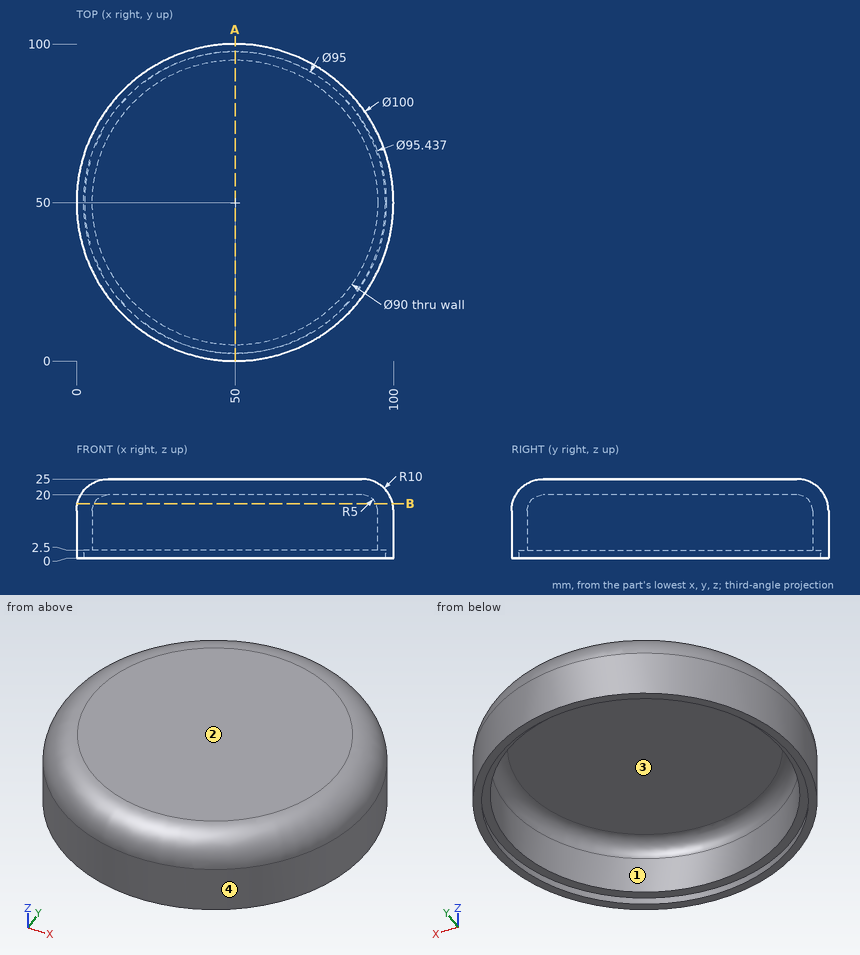
Verification items for this drawing (mm, ordinates from the low corner). Coordinates: 2 decimals unless noted, no trailing zeros. Order: outer loops, then holes, each group sorted by start corner. A loop starts at its lowest first (then second) coordinate and runs counter-clockwise, first axis right, second up. Notation, with made-up numbers: (11.5, 21) - (66.5, 21) arc R14 cw to (66.5, 27) - close; hole circle Ø8 at (-5, 87). An arc over 180 degrees is marked (long way). Use one line per item in the form item = value.
1. Section check A-A (x = 50). Record the boundary of the cut face in (y, z).
Here are the results:
outline = (0, 0) - (2.5, 0) - (2.28, 2.5) - (5, 2.5) - (5, 15) arc R5 cw to (10, 20) - (90, 20) arc R5 cw to (95, 15) - (95, 2.5) - (97.72, 2.5) - (97.5, 0) - (100, 0) - (100, 15) arc R10 ccw to (90, 25) - (10, 25) arc R10 ccw to (0, 15) - close
2. Scan lines: line 1 (Y direction, x = 50, z = 11.75); line 2 (Z direction, x = 75, y = 63.5); line 3 (Y direction, x = 68, z = 5.75). Record each from-to range of solid material in increasing order.
Here are the results:
line_1 = 0 to 5, 95 to 100
line_2 = 20 to 25
line_3 = 3.35 to 8.76, 91.24 to 96.65
3. Gauge pin test, flat ends, axial feed: pin 1 (2 mm diameter, centred on x = 70, y = 44.5, fed in from -Z); pin 2 (1 mm diameter, centred on x = 73.5, z = 5.5, fed in from -Y) (1 decimal); pin 3 (1.5 mm diameter, centred on x = 75.5, z = 20.5, fed in from -Y) (1 decimal). Record the tip position at first contact, or that the pin passes through.
Here are the results:
pin_1 = 20
pin_2 = 5.6
pin_3 = 8.2
4. Draft check along X on the marked faces 1, 2, 3 and 4. Enter one of: pulls with the +X half, pulls with the -X half, needs draft (parallel to the pull), parting line crosses it, or undercut.
Here are the results:
face_1 = undercut
face_2 = needs draft
face_3 = undercut
face_4 = parting line crosses it
5. Section check B-B (z = 17.25). Record the boundary of the cut face in (x, y) (1 decimal).
Here are the results:
outline = circle Ø99.5 at (50, 50); hole circle Ø88.9 at (50, 50)
